The model under review builds one solid part; all positions refer to its coordinate system, in mm. A direction names the side the tool comes from. Give positions to 0.01 mm unless a question says otherwise; leave off trailing zeros. Order: outer loops, then holes, each group sorted by start corner. A loop starts at its lowest first (then second) coordinate and runs counter-clockwise, first axis right, second up. Notation, with made-up numbers: (40.25, -4) - (94.25, -4) arc R16 cw to (94.25, 11) - close; hole circle Ø1 at (24.25, 66). An arc over 180 degrees is marked (long way). Write item = value, one per line. Start each with the question number.
1. For P1, Ø1.5, axis at y = 16.5, z = -0.5, coming from the +X side; P2, Ø1.5, axis at y = -11, z = 0, coming from the -X side; P3, Ø1, axis at y = 58, z = 1, coming from the -X side, all flat-tipped, find the tip position at first contact; note any pin that passes through.
2. We need section C-C, the plane x = -38. Give the boundary of the cut face in (y, z), and give its area (3 significant figures).
3. We need section B-B, the plane z = -0.8. State how many separate pieces and enclosed holes the cut face has, and give its area (3 significant figures).
4. Wall thickness on probe 1 along Y at (x, z) = (25.25, -0.4); probe 2 along X at (y, z) = (55.5, 1.4) (3 decimals); probe 3 along X at (y, z) = (28.5, -0.7): over which ranges is each line inside the solid? List them lowest first.
5. Machinability: for faces 1 (the flat face through (-47.25, -26, 0)), 2 (the flat face through (-55, -13.686, 0)), 3 (the flat face through (25.75, 45, 0)), which of the approach directions +Z, -Z, +X, -X, +Y, -Y give a long, thin tool a straight path to every point of the face, cutting with its end or side? Answer none if there is none.
6. Mouldability with a two-part tool opening along Y and no side actions: class faces 4 (the flat face through (6, 63.314, 0)), 5 (the flat face through (57.75, -26, 0)), 6 (the cylindrical face through (-10.661, 61.784, 0.137)) as pulls with the +Y half, pulls with the -Y half, needs draft (parallel to the pull), parting line crosses it, or undercut.
7. We need section A-A, the plane y = -24.5. Give the boundary of the cut face in (x, z).
from build123d import *

# Parameters (mm, degrees)
SKETCH1_R           = 0.15
BOSS_EXTRUDE1_DEPTH = 0.3175
SCALE1_SCALE        = 10


with BuildPart() as part:
    # Sketch1 → Boss-Extrude1 (new body)
    with BuildSketch(Plane.XY):
        Polygon((0, 0), (10.5, 0), (10.5, 1.5), (12, 1.5), (12, 2), (10.5, 2), (10.5, 2.5), (8.3, 2.5), (8.3, 6), (7.3, 6), (7.3, 9.7), (3.2, 9.7), (3.2, 6), (2.2, 6), (2.2, 2.5), (0, 2.5), (0, 2), (-1.5, 2), (-1.5, 1.5), (0, 1.5), align=None)
        with Locations((3.25, 0.5)):
            Circle(SKETCH1_R, mode=Mode.SUBTRACT)
        with Locations((7.25, 0.5)):
            Circle(SKETCH1_R, mode=Mode.SUBTRACT)
        with Locations((7.25, 4.5)):
            Circle(SKETCH1_R, mode=Mode.SUBTRACT)
        with Locations((3.25, 4.5)):
            Circle(SKETCH1_R, mode=Mode.SUBTRACT)
        with BuildLine():
            Line((3.8275, 9.382), (3.8275, 8.747))
            ThreePointArc((3.8275, 8.747), (3.6625, 8.582), (3.4975, 8.747))
            Line((3.4975, 8.747), (3.4975, 9.382))
            ThreePointArc((3.4975, 9.382), (3.6625, 9.547), (3.8275, 9.382))
        make_face(mode=Mode.SUBTRACT)
        with BuildLine():
            Line((6.6725, 9.382), (6.6725, 8.747))
            ThreePointArc((6.6725, 8.747), (6.8375, 8.582), (7.0025, 8.747))
            Line((7.0025, 8.747), (7.0025, 9.382))
            ThreePointArc((7.0025, 9.382), (6.8375, 9.547), (6.6725, 9.382))
        make_face(mode=Mode.SUBTRACT)
        with BuildLine():
            Line((3.4025, 6.3975), (3.4025, 6.6515))
            ThreePointArc((3.4025, 6.6515), (3.6625, 6.9115), (3.9225, 6.6515))
            Line((3.9225, 6.6515), (3.9225, 6.3975))
            ThreePointArc((3.9225, 6.3975), (3.6625, 6.1375), (3.4025, 6.3975))
        make_face(mode=Mode.SUBTRACT)
        with BuildLine():
            Line((7.0975, 6.3975), (7.0975, 6.6515))
            ThreePointArc((7.0975, 6.6515), (6.8375, 6.9115), (6.5775, 6.6515))
            Line((6.5775, 6.6515), (6.5775, 6.3975))
            ThreePointArc((6.5775, 6.3975), (6.8375, 6.1375), (7.0975, 6.3975))
        make_face(mode=Mode.SUBTRACT)
    extrude(amount=BOSS_EXTRUDE1_DEPTH)


with BuildPart() as part_1:
    # Scale1: scaled about (5.25, 3.742866372, 0.15875)
    add(part.part.scale(SCALE1_SCALE).moved(Location((-47.25, -33.685797348, -1.42875))))


solid = part_1.part
Model answer:
q1.P1 = 35.75
q1.P2 = -47.25
q1.P3 = -15.25
q2.outline = (-33.69, -1.43) - (-8.69, -1.43) - (-8.69, 1.75) - (-33.69, 1.75) - close
q2.area = 79.4 mm2
q3.separate_pieces = 1
q3.enclosed_holes = 8
q3.area = 6,270 mm2
q4.probe_1 = -33.69 to -30.19, -27.19 to 9.81, 12.81 to 63.31
q4.probe_2 = -15.25 to -12.275, -8.975 to 19.475, 22.775 to 25.75
q4.probe_3 = -15.25 to -12.51, -8.74 to 19.24, 23.01 to 25.75
q5.face_1 = +Z, -Z, -X, -Y
q5.face_2 = +Z, -Z, -X, +Y
q5.face_3 = +Z, -Z, +X, +Y
q6.face_4 = pulls with the +Y half
q6.face_5 = needs draft
q6.face_6 = undercut
q7.outline = (-47.25, -1.43) - (57.75, -1.43) - (57.75, 1.75) - (-47.25, 1.75) - close
